Answer from the drawing. Dimensions are ordinates in mm from the lowest x, y and z of the part. A direction names the side the tool comes from. Give positions to 0.01 mm unless a question says otherwise; leave off trailing zeros. Write each loop counter-clockwise with the first axis right and the second up, starting at its lowest first coordinate (ties: lowest second). Pieces come first, ordered by that corner, then holes. Notation, with made-up numbers: M -26,42.5 L 9,42.5 A33 ccw 9,73.5 Z; hole C -28,70 d6. An arc over 180 degrees is marked long. Put each result on its own line as item: value.
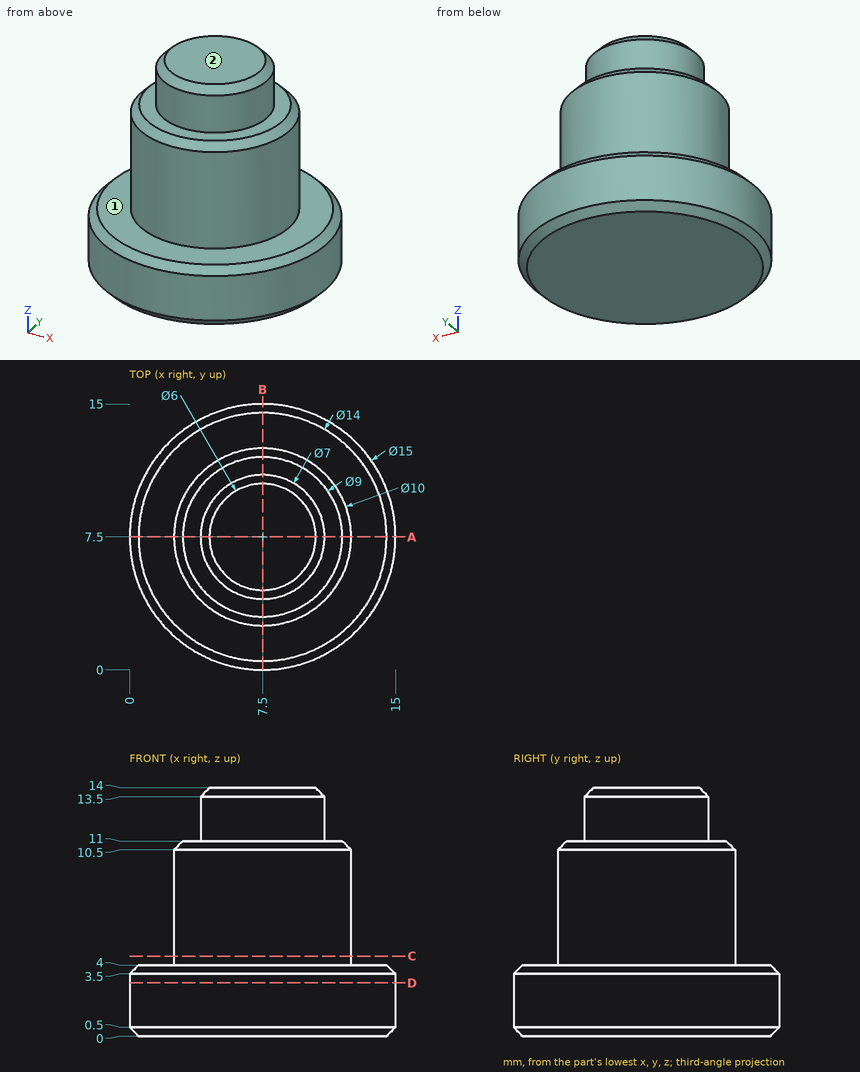
(1) Which of the six approach directions +Z, -Z, +X, -X, +Y, -Y give full straight-line access (tool end or side, diameter ignored) to the marked faces 1 and 2?
Result:
face 1: +Z
face 2: +Z, +X, -X, +Y, -Y
(2) Given pin 1 Ø6 at (x, z) = (6, 10) entering from -Y; pin 2 Ø2 at (y, z) = (9.5, 10.5) entering from +X; pin 3 Ø2 at (x, z) = (4.5, 12.5) entering from -Y, each flat-ended and moving along its own axis, determine where each tip first touches the part or whether it passes through.
Result:
pin 1: stops at y = 2.5
pin 2: stops at x = 12.4
pin 3: stops at y = 4.63
(3) Section C-C on z = 4.5 is taken. Determine the outline of the cut face in (x, y).
Result:
outline: C 7.5,7.5 d10
(4) Section A-A on y = 7.5 is taken. Determine the outline of the cut face in (x, z), and give its area (3 significant figures).
Result:
outline: M 0,0.5 L 0.5,0 L 14.5,0 L 15,0.5 L 15,3.5 L 14.5,4 L 12.5,4 L 12.5,10.5 L 12,11 L 11,11 L 11,13.5 L 10.5,14 L 4.5,14 L 4,13.5 L 4,11 L 3,11 L 2.5,10.5 L 2.5,4 L 0.5,4 L 0,3.5 Z
area: 150 mm²
(5) Section D-D on z = 3 is taken. Determine the outline of the cut face in (x, y).
Result:
outline: C 7.5,7.5 d15
(6) Straight lines are drawn through the part: line 1 along Z through (x, y) = (2.75, 12.5); line 2 along X through (y, z) = (3.5, 5.75); line 3 along Z through (x, y) = (8.5, 3.5). For each, find the intervals that lie inside material, in ascending order. Write a range as from..to.
Result:
line 1: z = 0..4
line 2: x = 4.5..10.5
line 3: z = 0..11
